Check sheet for the modelled part. Datum: model origin and axes. Units: mm. Face numbers are marked on the shaded views. A direction names the side the tool comes from. Coordinates: 2 decimals unless noted, no trailing zeros. Loops run counter-clockwise (first coordinate to the right, second up) from the corner with the lowest first, then second, coordinate; pieces in that order, holes last.
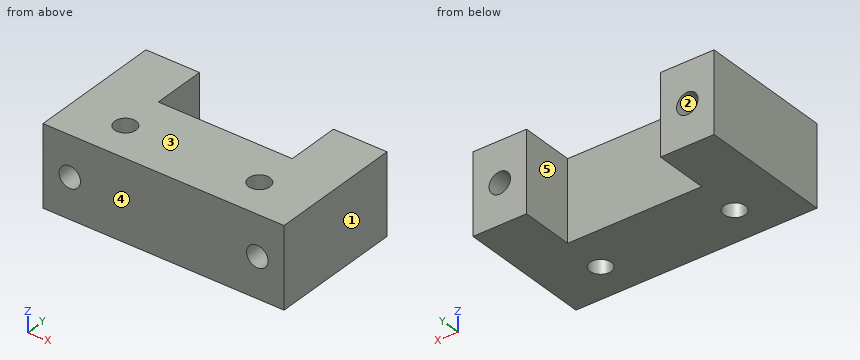
Autodesk Inventor part; units mm, degrees
ref_plane "YZ Plane" through (0, 0, 0) normal (1, 0, 0) x (0, 1, 0)
ref_plane "XZ Plane" through (0, 0, 0) normal (0, 1, 0) x (-1, 0, 0)
ref_plane "XY Plane" through (0, 0, 0) normal (0, 0, 1) x (1, 0, 0)
sketch "Sketch1" plane through (0, 0, 0) normal (0, 0, 1) x (1, 0, 0)
  line L0 (-22.5, 0) -> (22.5, 0)
  line L1 (22.5, 0) -> (22.5, 25)
  line L2 (22.5, 25) -> (12.5, 25)
  line L3 (12.5, 25) -> (12.5, 15)
  line L4 (12.5, 15) -> (-12.5, 15)
  line L5 (-12.5, 15) -> (-12.5, 25)
  line L6 (-12.5, 25) -> (-22.5, 25)
  line L7 (-22.5, 25) -> (-22.5, 0)
  point P0 (0, 0)
  point P1 (0, 0)
  dimension "d0" = 45
  dimension "d1" = 25
  dimension "d2" = 10
  dimension "d3" = 10
extrude "Extrusion1" add sketch "Sketch1" along normal mid plane 15
sketch "Sketch2" plane through (12.5, 25, -7.5) normal (0, 1, 0) x (1, 0, 0)
  line L0 (0, 0) -> (10, 0)
  line L1 (0, 0) -> (0, -15)
  line L2 (10, -15) -> (0, -15)
  line L3 (10, 0) -> (10, -15)
  line L4 (-35, 0) -> (-25, 0)
  line L5 (-35, 0) -> (-35, -15)
  line L6 (-25, -15) -> (-35, -15)
  line L7 (-25, 0) -> (-25, -15)
  line L8 (-25, 0) -> (-25, -15)
  line L9 (5, -7.5) -> (-30, -7.5)
  point P0 (-12.5, -7.5)
  point P1 (-12.5, -7.5)
  dimension "d6" = 35
hole "Hole1" at (17.5, 25, 0) at (-17.5, 25, 0) direction (0, -1, 0) diameter 4 end through all
sketch "Sketch3" plane through (0, 0, 7.5) normal (0, 0, 1) x (1, 0, 0)
  line L0 (12.5, 7) -> (-12.5, 7) construction
  line L1 (0, 0) -> (0, 14) construction
  line L2 (12.5, 15) -> (-12.5, 15)
  point P0 (0, 7)
  dimension "d14" = 8
  dimension "d15" = 25
hole "Hole2" at (12.5, 7, 7.5) at (-12.5, 7, 7.5) direction (0, 0, -1) diameter 4 end through all
properties part number "sujetador inferior"
1) Depth check by flat-ended pin: pin 1 (3 mm diameter, centred on x = -17.5, z = 0, fed in from -Y); pin 2 (4 mm diameter, centred on x = -5, z = -5, fed in from +Y). Enter the tip coordinate at first touch or a pass-through.
Answer sheet:
pin 1: passes through
pin 2: stops at y = 15
2) Section check B-B on z = 0. Enter the section's corners in (x, y).
Answer sheet:
outline: (-22.5, 0) - (-19.5, 0) - (-19.5, 25) - (-22.5, 25) - close; (-15.5, 0) - (15.5, 0) - (15.5, 25) - (12.5, 25) - (12.5, 15) - (-12.5, 15) - (-12.5, 25) - (-15.5, 25) - close; (19.5, 0) - (22.5, 0) - (22.5, 25) - (19.5, 25) - close; hole circle Ø4 at (-12.5, 7); hole circle Ø4 at (12.5, 7)
3) Section check C-C on z = -6.5. Enter the section's corners in (x, y), plus the area to 3 significant figures.
Answer sheet:
outline: (-22.5, 0) - (22.5, 0) - (22.5, 25) - (12.5, 25) - (12.5, 15) - (-12.5, 15) - (-12.5, 25) - (-22.5, 25) - close; hole circle Ø4 at (-12.5, 7); hole circle Ø4 at (12.5, 7)
area: 850 mm2
4) Set-up check for the marked faces 4 and 5: record each of +Z, -Z, +X, -X, +Y, -Y from which the full face is reachable in a straight line by a thin tool's end or side.
Answer sheet:
face 4: +Z, -Z, +X, -X, -Y
face 5: +Z, -Z, +Y
5) Mould release check, pull along Z, two halves, no side actions. Record for the marked faces 1, 2 and 3: +Z half, -Z half, draft (parallel to the pull), parting line (faces both ways), or undercut.
Answer sheet:
face 1: draft
face 2: undercut
face 3: +Z half
6) Section check A-A on y = 7. Enter the section's corners in (x, z), plus the area to 3 significant figures.
Answer sheet:
outline: (-22.5, -7.5) - (-14.5, -7.5) - (-14.5, 7.5) - (-22.5, 7.5) - close; (-10.5, -7.5) - (10.5, -7.5) - (10.5, 7.5) - (-10.5, 7.5) - close; (14.5, -7.5) - (22.5, -7.5) - (22.5, 7.5) - (14.5, 7.5) - close; hole circle Ø4 at (-17.5, 0); hole circle Ø4 at (17.5, 0)
area: 530 mm2
7) Scan lines: line 1 (X direction, y = 7, z = -2.5); line 2 (X direction, y = 14.5, z = 0); line 3 (X direction, y = 15.75, z = 0). Record each from-to range of solid material in increasing order.
Answer sheet:
line 1: x = -22.5 to -14.5, -10.5 to 10.5, 14.5 to 22.5
line 2: x = -22.5 to -19.5, -15.5 to 15.5, 19.5 to 22.5
line 3: x = -22.5 to -19.5, -15.5 to -12.5, 12.5 to 15.5, 19.5 to 22.5
8) Section check D-D on y = 21.5. Enter the section's corners in (x, z).
Answer sheet:
outline: (-22.5, -7.5) - (-12.5, -7.5) - (-12.5, 7.5) - (-22.5, 7.5) - close; (12.5, -7.5) - (22.5, -7.5) - (22.5, 7.5) - (12.5, 7.5) - close; hole circle Ø4 at (-17.5, 0); hole circle Ø4 at (17.5, 0)
